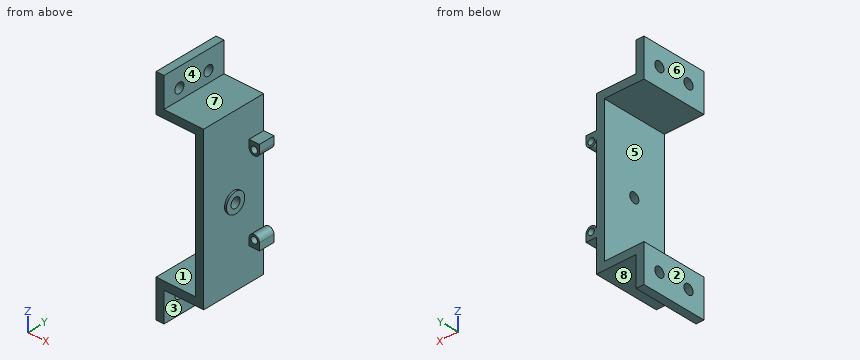
Autodesk Inventor part; units mm, degrees
ref_plane "YZ Plane" through (0, 0, 0) normal (1, 0, 0) x (0, 1, 0)
ref_plane "XZ Plane" through (0, 0, 0) normal (0, 1, 0) x (-1, 0, 0)
ref_plane "XY Plane" through (0, 0, 0) normal (0, 0, 1) x (1, 0, 0)
sketch "Sketch1" plane through (0, 0, 0) normal (1, 0, 0) x (0, 1, 0)
  line L0 (0, 0) -> (33, 0)
  line L1 (33, 0) -> (33, 19)
  line L2 (33, 19) -> (0, 19)
  line L3 (0, 19) -> (0, 0)
  circle A0 centre (24.5, 9.5) radius 2.5
  circle A1 centre (8.5, 9.5) radius 2.5
  dimension "d0" = 33
  dimension "d1" = 19
  dimension "d2" = 33
  dimension "d3" = 19
  dimension "d6" = 5
  dimension "d8" = 5
extrude "Extrusion1" add sketch "Sketch1" along normal blind 4
sketch "Sketch2" plane through (0, 33, 19) normal (0, 1, 0) x (1, 0, 0)
  line L0 (0, 19) -> (4, 19)
  line L1 (0, 19) -> (24, 19)
  line L2 (24, 19) -> (24, 15)
  line L3 (24, 15) -> (0, 15)
  line L4 (0, 19) -> (0, 0)
  line L5 (0, 15) -> (0, 19)
  dimension "d11" = 24
  dimension "d12" = 4
  dimension "d13" = 24
extrude "Extrusion2" add sketch "Sketch2" against normal blind 33
sketch "Sketch3" plane through (0, 33, 19) normal (0, 1, 0) x (1, 0, 0)
  line L0 (4, 15) -> (24, 15)
  line L1 (24, 15) -> (24, 95)
  line L2 (24, 15) -> (20, 15)
  line L3 (20, 15) -> (20, 95)
  line L4 (20, 95) -> (24, 95)
  point P0 (0, 19)
  dimension "d16" = 80
  dimension "d17" = 4
  dimension "d18" = 80
  dimension "d19" = 4
extrude "Extrusion3" add sketch "Sketch3" against normal blind 33
sketch "Sketch4" plane through (0, 33, 19) normal (0, 1, 0) x (1, 0, 0)
  line L0 (24, 95) -> (20, 95)
  line L1 (24, 95) -> (0, 95)
  line L2 (0, 95) -> (0, 91)
  line L3 (0, 91) -> (24, 91)
  line L4 (24, 15) -> (24, 95)
  line L5 (24, 91) -> (24, 95)
  point P0 (0, 19)
  dimension "d22" = 24
  dimension "d23" = 4
  dimension "d24" = 24
  dimension "d25" = 4
extrude "Extrusion4" add sketch "Sketch4" against normal blind 33
sketch "Sketch5" plane through (0, 33, 19) normal (0, 1, 0) x (1, 0, 0)
  line L0 (0, 91) -> (0, 110)
  line L1 (0, 110) -> (4, 110)
  line L2 (4, 110) -> (4, 91)
  line L3 (20, 91) -> (0, 91)
  line L4 (4, 91) -> (0, 91)
  point P0 (0, 19)
  dimension "d28" = 19
  dimension "d29" = 4
  dimension "d30" = 19
  dimension "d31" = 4
extrude "Extrusion5" add sketch "Sketch5" against normal blind 33
sketch "Sketch6" plane through (4, 33, -76) normal (1, 0, 0) x (0, 0, -1)
  line L0 (15, 0) -> (-4, 0)
  circle A0 centre (5.5, -8.5) radius 2.5
  circle A1 centre (5.5, -24.5) radius 2.5
  point P0 (-76, -33)
  dimension "d36" = 5
  dimension "d38" = 5
hole "Hole1" at (4, 24.5, -81.5) at (4, 8.5, -81.5) direction (-1, 0, 0) diameter 5 end through all both
sketch "Sketch7" plane through (24, 0, 4) normal (1, 0, 0) x (0, 0, -1)
  line L0 (0, 33) -> (80, 33)
  circle A0 centre (40, 16.5) radius 5
  circle A1 centre (40, 16.5) radius 2.5
  point P0 (4, 0)
  point P1 (0, 0)
  dimension "d46" = 10
  dimension "d47" = 5
hole "Hole2" at (24, 16.5, -36) direction (-1, 0, 0) diameter 5 end through all both
extrude "Extrusion6" add sketch "Sketch7" along normal blind 1
sketch "Sketch8" plane through (0, 33, 19) normal (0, 1, 0) x (1, 0, 0)
  line L0 (24, 31.4) -> (29.2, 31.4)
  line L1 (29.2, 31.4) -> (29.2, 35)
  line L2 (26.6, 37.6) -> (26.6, 37.6)
  line L3 (24, 35) -> (24, 31.4)
  arc A0 (26.6, 37.6) -> (24, 35) centre (26.6, 35) ccw
  arc A1 (29.2, 35) -> (26.6, 37.6) centre (26.6, 35) ccw
  circle A2 centre (26.6, 35) radius 1.6
  point P0 (0, 19)
  point P1 (24, 15)
  point P2 (29.2, 37.6)
  point P3 (24, 37.6)
  dimension "d58" = 5.2
  dimension "d59" = 6.2
  dimension "d60" = 5.2
  dimension "d61" = 6.2
  dimension "d62" = 2.6
  dimension "d63" = 3.2
extrude "Extrusion7" add sketch "Sketch8" against normal blind 8
sketch "Sketch9" plane through (0, 33, 19) normal (0, 1, 0) x (1, 0, 0)
  line L0 (24, 95) -> (4, 95)
  line L1 (24, 95) -> (24, 15)
  line L2 (24, 78.6) -> (29.2, 78.6)
  line L3 (29.2, 78.6) -> (29.2, 75)
  line L4 (26.6, 72.4) -> (26.6, 72.4)
  line L5 (24, 75) -> (24, 78.6)
  arc A0 (26.6, 72.4) -> (29.2, 75) centre (26.6, 75) ccw
  arc A1 (24, 75) -> (26.6, 72.4) centre (26.6, 75) ccw
  circle A2 centre (26.6, 75) radius 1.6
  point P0 (0, 19)
  point P1 (29.2, 72.4)
  point P2 (24, 72.4)
  dimension "d67" = 5.2
  dimension "d68" = 6.2
  dimension "d69" = 5.2
  dimension "d70" = 6.2
  dimension "d71" = 2.6
  dimension "d72" = 3.2
extrude "Extrusion8" add sketch "Sketch9" against normal blind 8
Source: CAD feature listing. Evaluate the final solid. Frame: model axes, mm. Face numbers are marked on the shaded views. A direction names the side the tool comes from. Give positions to 0.01 mm unless a question says otherwise; leave off trailing zeros. Write each loop counter-clockwise with the first axis right and the second up, starting at its lowest first coordinate (ties: lowest second). Pieces come first, ordered by that corner, then holes.
1. Section query D-D (x = 22). Return the cut outline in (y, z).
2. First-contact query: pin 1 (1.5 mm diameter, centred on x = 16, y = 29.5, fed in from +Z); pin 2 (5.5 mm diameter, centred on x = 27, z = -56.5, fed in from -Y); pin 3 (10 mm diameter, centred on x = 12.5, y = 18, fed in from -Z). Flat tips, straight axial feed; report the tip coordinate or a pass-through.
3. Section query B-B (z = -81.5). Return the cut outline in (x, y).
4. Access query for the marked faces 1, 2, 3 and 4. Directions: +Z, -Z, +X, -X, +Y, -Y. A direction counts if a zero-diameter tool reaches every point of the face in a straight line with its end or side. Return the directions, or none.
5. Material intervals for line 1 along Z through (x, y) = (3, 24.5); line 2 along Z through (x, y) = (12.5, 4.5); line 3 along Z through (x, y) = (26.6, 27.5), sorted ascending.
6. Section query C-C (x = 26.6). Return the cut outline in (y, z).
7. Pull-direction query (Z, two-part tool) for the marked faces 5, 6, 7 and 8; classes: +Z half, -Z half, draft (parallel to the pull), parting line (faces both ways), or undercut.
8. Section query A-A (x = 5.5). Return the cut outline in (y, z).
Output values:
1. outline: (0, -76) - (33, -76) - (33, 4) - (0, 4) - close; hole circle Ø5 at (16.5, -36)
2. pin 1: stops at z = 4
2. pin 2: stops at y = 25
2. pin 3: stops at z = -76
3. outline: (0, 0) - (4, 0) - (4, 6) - (0, 6) - close; (0, 11) - (4, 11) - (4, 22) - (0, 22) - close; (0, 27) - (4, 27) - (4, 33) - (0, 33) - close
4. face 1: -X, +Y, -Y
4. face 2: +Z, -Z, -X, +Y, -Y
4. face 3: -Z, +X, +Y, -Y
4. face 4: +Z, +X, +Y, -Y
5. line 1: z = -91 to -84, -79 to -72, 0 to 7, 12 to 19
5. line 2: z = -76 to -72, 0 to 4
5. line 3: z = -59.6 to -57.6, -54.4 to -53.4, -18.6 to -17.6, -14.4 to -12.4
6. outline: (25, -59.6) - (33, -59.6) - (33, -57.6) - (25, -57.6) - close; (25, -54.4) - (33, -54.4) - (33, -53.4) - (25, -53.4) - close; (25, -18.6) - (33, -18.6) - (33, -17.6) - (25, -17.6) - close; (25, -14.4) - (33, -14.4) - (33, -12.4) - (25, -12.4) - close
7. face 5: undercut
7. face 6: draft
7. face 7: +Z half
7. face 8: -Z half
8. outline: (0, -76) - (33, -76) - (33, -72) - (0, -72) - close; (0, 0) - (33, 0) - (33, 4) - (0, 4) - close
